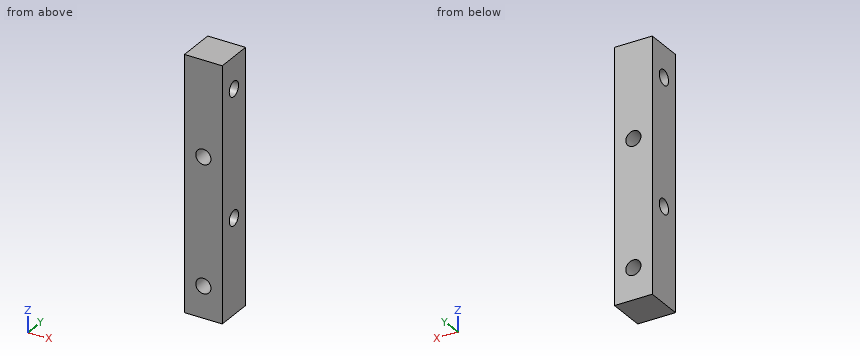
from build123d import *

# Parameters (mm, degrees)
SKETCH_1_W          = 6
SKETCH_1_H          = 6
EXTRUDE_1_DEPTH     = 40
SKETCH_2_R          = 1.2
CUT_EXTRUDE_1_DEPTH = 50
SKETCH_3_R          = 1.2
CUT_EXTRUDE_2_DEPTH = 50


with BuildPart() as part:
    # 草图1 → 凸台-拉伸1 (new body)
    with BuildSketch(Plane.XY):
        with Locations((3, 3)):
            Rectangle(SKETCH_1_W, SKETCH_1_H)
    extrude(amount=EXTRUDE_1_DEPTH)

    # 草图2 → 切除-拉伸1 (cut)
    with BuildSketch(Plane(origin=(0, 6, 0), x_dir=(1, 0, 0), z_dir=(0, 1, 0))):
        with Locations((3, -5)):
            Circle(SKETCH_2_R)
        with Locations((3, -25)):
            Circle(SKETCH_2_R)
    extrude(amount=-CUT_EXTRUDE_1_DEPTH, mode=Mode.SUBTRACT)

    # 草图3 → 切除-拉伸2 (cut)
    with BuildSketch(Plane.ZY):
        with Locations((35, 3)):
            Circle(SKETCH_3_R)
        with Locations((15, 3)):
            Circle(SKETCH_3_R)
    extrude(amount=-CUT_EXTRUDE_2_DEPTH, mode=Mode.SUBTRACT)


solid = part.part
Model file for the job. Use its own axes, mm. Give positions to 0.01 mm unless a question says otherwise; leave off trailing zeros. Loops run counter-clockwise (first coordinate to the right, second up) from the corner with the lowest first, then second, coordinate; pieces in that order, holes last. Notation, with made-up numbers: (-37, 21) -> (13, 21) arc R25 ccw to (13, 51) -> close; hole circle Ø10 at (-23.75, 57.25). An arc over 180 degrees is marked (long way). Use a Markdown table: item, result. Add a question column.
(1) Slice it at B-B on z = 25. List the corners of the cut face in (x, y), and give its area (3 significant figures).
(2) Wall check: line 1 along Z through (x, y) = (3, 4.25); line 2 along X through (y, z) = (2.4, 5); line 3 along Z through (x, y) = (2.2, 2.4). Give the ranges that are in metal, low to high.
(3) Slice it at D-D on x = 5.5. List the corners of the cut face in (y, z).
(4) Slice it at A-A on x = 3. List the corners of the cut face in (y, z), and give its area (3 significant figures).
(5) Slice it at C-C on y = 3.55. List the corners of the cut face in (x, z), and give its area (3 significant figures).
Filled sheet:
| question | item | result |
|---|---|---|
| 1 | outline | (0, 0) -> (1.8, 0) -> (1.8, 6) -> (0, 6) -> close; (4.2, 0) -> (6, 0) -> (6, 6) -> (4.2, 6) -> close |
| 1 | area | 21.6 mm2 |
| 2 | line 1 | 0 to 3.8, 6.2 to 23.8, 26.2 to 40 |
| 2 | line 2 | 0 to 1.8, 4.2 to 6 |
| 2 | line 3 | 0 to 4.11, 5.89 to 13.96, 16.04 to 24.11, 25.89 to 33.96, 36.04 to 40 |
| 3 | outline | (0, 0) -> (6, 0) -> (6, 40) -> (0, 40) -> close; hole circle Ø2.4 at (3, 15); hole circle Ø2.4 at (3, 35) |
| 4 | outline | (0, 0) -> (6, 0) -> (6, 3.8) -> (0, 3.8) -> close; (0, 6.2) -> (6, 6.2) -> (6, 23.8) -> (0, 23.8) -> close; (0, 26.2) -> (6, 26.2) -> (6, 40) -> (0, 40) -> close; hole circle Ø2.4 at (3, 15); hole circle Ø2.4 at (3, 35) |
| 4 | area | 202 mm2 |
| 5 | outline | (0, 0) -> (6, 0) -> (6, 13.93) -> (0, 13.93) -> close; (0, 16.07) -> (6, 16.07) -> (6, 33.93) -> (0, 33.93) -> close; (0, 36.07) -> (6, 36.07) -> (6, 40) -> (0, 40) -> close; hole circle Ø2.4 at (3, 5); hole circle Ø2.4 at (3, 25) |
| 5 | area | 205 mm2 |
